Geometry: final body of the model. Coordinates: model frame, mm. Give positions to 0.01 mm unless a question says otherwise; leave off trailing zeros. Use a Markdown table: item, result. Add a question column.
(1) Material intervals for L1, parallel to Y at x = -6.5, z = 308.5; L2, parallel to Y at x = 8.5, z = 583.5 (3 decimals); L3, parallel to X at y = 5, z = 223, sorted ascending.
(2) Pin query (flat end, axial travel): pin 1 Ø2 at (y, z) = (-1, 468.5) entering from -X; pin 2 Ø2 at (x, z) = (1.5, 465) entering from -Y; pin 3 Ø3 at (y, z) = (1, 596.5) entering from +X; pin 4 Ø6 at (x, y) = (-1, -8) entering from +Z. Return the tip coordinate at first contact, or that it passes through.
(3) Cut plane A-A (z = 658). State how many separate pieces and enclosed holes the cut face has, plus the area to 3 significant figures.
```python
from build123d import *

# Parameters (mm, degrees)
BOSS_EXTRU_1_DEPTH  = 1000
SYM_TRIE6_OUTLINE_R = 2.1
SYM_TRIE6_DEPTH     = 1000


# Read off the part's stored shape, not the designer's step: Symétrie6
with BuildPart() as part:
    # Esquisse1 → Boss.-Extru.1 (new body)
    with BuildSketch(Plane.XY):
        with BuildLine():
            Line((-9.5, 10), (-4.58, 10))
            Line((-4.58, 10), (-3.125, 8.545))
            Line((-3.125, 8.545), (-3.125, 8.2))
            Line((-3.125, 8.2), (-5.5, 8.2))
            Line((-5.5, 8.2), (-5.5, 6.560660172))
            Line((-5.5, 6.560660172), (-2.839339828, 3.9))
            Line((-2.839339828, 3.9), (-0.21, 3.9))
            Line((-0.21, 3.9), (0, 3.69))
            Line((0, 3.69), (0, 2.1))
            ThreePointArc((0, 2.1), (-2.1, 0), (0, -2.1))
            Line((0, -2.1), (0, -3.69))
            Line((0, -3.69), (-0.21, -3.9))
            Line((-0.21, -3.9), (-2.839339828, -3.9))
            Line((-2.839339828, -3.9), (-6.239339828, -7.3))
            Line((-6.239339828, -7.3), (-8.2, -7.3))
            Line((-8.2, -7.3), (-8.2, -10))
            Line((-8.2, -10), (-10, -10))
            Line((-10, -10), (-10, -4.58))
            Line((-10, -4.58), (-8.545, -3.125))
            Line((-8.545, -3.125), (-8.2, -3.125))
            Line((-8.2, -3.125), (-8.2, -5.5))
            Line((-8.2, -5.5), (-6.560660172, -5.5))
            Line((-6.560660172, -5.5), (-3.9, -2.839339828))
            Line((-3.9, -2.839339828), (-3.9, -0.21))
            Line((-3.9, -0.21), (-3.69, 0))
            Line((-3.69, 0), (-3.9, 0.21))
            Line((-3.9, 0.21), (-3.9, 2.839339828))
            Line((-3.9, 2.839339828), (-6.560660172, 5.5))
            Line((-6.560660172, 5.5), (-8.2, 5.5))
            Line((-8.2, 5.5), (-8.2, 3.125))
            Line((-8.2, 3.125), (-8.545, 3.125))
            Line((-8.545, 3.125), (-10, 4.58))
            Line((-10, 4.58), (-10, 9.5))
            ThreePointArc((-10, 9.5), (-9.853553391, 9.853553391), (-9.5, 10))
        make_face()
    boss_extru_1 = extrude(amount=BOSS_EXTRU_1_DEPTH)

    # Symétrie1: Boss.-Extru.1 across Right Plane
    add(boss_extru_1.mirror(Plane(origin=(0, 0, 0), x_dir=(0, 0, -1), z_dir=(1, 0, 0))))

    # Symétrie6 outline → Symétrie6 (add)
    with BuildSketch(Plane.XY):
        with BuildLine():
            Line((-3.9, -17.160660172), (-3.9, -19.79))
            Line((-3.9, -19.79), (-3.69, -20))
            Line((-3.69, -20), (-3.9, -20.21))
            Line((-3.9, -20.21), (-3.9, -22.839339828))
            Line((-3.9, -22.839339828), (-6.560660172, -25.5))
            Line((-6.560660172, -25.5), (-8.2, -25.5))
            Line((-8.2, -25.5), (-8.2, -23.125))
            Line((-8.2, -23.125), (-8.545, -23.125))
            Line((-8.545, -23.125), (-10, -24.58))
            Line((-10, -24.58), (-10, -29.5))
            ThreePointArc((-10, -29.5), (-9.853553391, -29.853553391), (-9.5, -30))
            Line((-9.5, -30), (-4.58, -30))
            Line((-4.58, -30), (-3.125, -28.545))
            Line((-3.125, -28.545), (-3.125, -28.2))
            Line((-3.125, -28.2), (-5.5, -28.2))
            Line((-5.5, -28.2), (-5.5, -26.560660172))
            Line((-5.5, -26.560660172), (-2.839339828, -23.9))
            Line((-2.839339828, -23.9), (-0.21, -23.9))
            Line((-0.21, -23.9), (0, -23.69))
            Line((0, -23.69), (0.21, -23.9))
            Line((0.21, -23.9), (2.839339828, -23.9))
            Line((2.839339828, -23.9), (5.5, -26.560660172))
            Line((5.5, -26.560660172), (5.5, -28.2))
            Line((5.5, -28.2), (3.125, -28.2))
            Line((3.125, -28.2), (3.125, -28.545))
            Line((3.125, -28.545), (4.58, -30))
            Line((4.58, -30), (9.5, -30))
            ThreePointArc((9.5, -30), (9.853553391, -29.853553391), (10, -29.5))
            Line((10, -29.5), (10, -24.58))
            Line((10, -24.58), (8.545, -23.125))
            Line((8.545, -23.125), (8.2, -23.125))
            Line((8.2, -23.125), (8.2, -25.5))
            Line((8.2, -25.5), (6.560660172, -25.5))
            Line((6.560660172, -25.5), (3.9, -22.839339828))
            Line((3.9, -22.839339828), (3.9, -20.21))
            Line((3.9, -20.21), (3.69, -20))
            Line((3.69, -20), (3.9, -19.79))
            Line((3.9, -19.79), (3.9, -17.160660172))
            Line((3.9, -17.160660172), (6.560660172, -14.5))
            Line((6.560660172, -14.5), (8.2, -14.5))
            Line((8.2, -14.5), (8.2, -16.875))
            Line((8.2, -16.875), (8.545, -16.875))
            Line((8.545, -16.875), (10, -15.42))
            Line((10, -15.42), (10, -10))
            Line((10, -10), (8.2, -10))
            Line((8.2, -10), (8.2, -12.7))
            Line((8.2, -12.7), (6.239339828, -12.7))
            Line((6.239339828, -12.7), (2.839339828, -16.1))
            Line((2.839339828, -16.1), (0.21, -16.1))
            Line((0.21, -16.1), (0, -16.31))
            Line((0, -16.31), (-0.21, -16.1))
            Line((-0.21, -16.1), (-2.839339828, -16.1))
            Line((-2.839339828, -16.1), (-6.239339828, -12.7))
            Line((-6.239339828, -12.7), (-8.2, -12.7))
            Line((-8.2, -12.7), (-8.2, -10))
            Line((-8.2, -10), (-10, -10))
            Line((-10, -10), (-10, -15.42))
            Line((-10, -15.42), (-8.545, -16.875))
            Line((-8.545, -16.875), (-8.2, -16.875))
            Line((-8.2, -16.875), (-8.2, -14.5))
            Line((-8.2, -14.5), (-6.560660172, -14.5))
            Line((-6.560660172, -14.5), (-3.9, -17.160660172))
        make_face()
        with Locations((0, -20)):
            Circle(SYM_TRIE6_OUTLINE_R, mode=Mode.SUBTRACT)
    extrude(amount=SYM_TRIE6_DEPTH)


solid = part.part
```
Answer list:
| question | item | result |
|---|---|---|
| 1 | L1 | -30 to -25.44, -14.56 to -12.7, -7.3 to -5.44, 5.44 to 10 |
| 1 | L2 | -30 to -23.125, -16.875 to -3.125, 3.125 to 10 |
| 1 | L3 | -10 to -8.2, -6.06 to -3.94, 3.94 to 6.06, 8.2 to 10 |
| 2 | pin 1 | x = -3.9 |
| 2 | pin 2 | y = -23.9 |
| 2 | pin 3 | x = 3.9 |
| 2 | pin 4 | through |
| 3 | separate pieces | 1 |
| 3 | enclosed holes | 3 |
| 3 | area | 300 mm² |
